```python
from build123d import *

# Parameters (mm, degrees)
F1_DEPTH       = 76.2
F1_DEPTH_BACK  = 76.2
F3_D           = 3.683
F3_CSINK_D     = 5.588
F3_CSINK_ANGLE = 100


with BuildPart() as f1:
    # F0 (on Front) → F1 (new body, two sides)
    with BuildSketch(Plane.XZ) as f1_sk:
        with BuildLine():
            Line((0, 1.0668), (0, 0))
            Line((0, 0), (127, 0))
            ThreePointArc((127, 0), (135.980256, -3.719744), (139.7, -12.7))
            Line((139.7, -12.7), (140.7668, -12.7))
            ThreePointArc((140.7668, -12.7), (136.734598, -2.965402), (127, 1.0668))
            Line((127, 1.0668), (0, 1.0668))
        make_face()
    extrude(amount=F1_DEPTH)
    extrude(f1_sk.sketch, amount=-F1_DEPTH_BACK)

    # F3 (through all)
    with Locations(Plane(origin=(0, 0, 0), x_dir=(1, 0, 0), z_dir=(0, 0, -1))):
        with Locations((63.5, 42.8625), (63.5, 0), (63.5, -42.8625)):
            CounterSinkHole(F3_D / 2, F3_CSINK_D / 2, counter_sink_angle=F3_CSINK_ANGLE)


solid = f1.part
```
Can you work these out from the model? Positions are in its coordinate system, mm. A direction names the side the tool comes from. Give positions to 0.01 mm unless a question says otherwise; leave off trailing zeros. Write each loop counter-clockwise with the first axis right and the second up, starting at its lowest first coordinate (ties: lowest second). Pieces come first, ordered by that corner, then holes. Notation, with made-up numbers: (-13, 79.5) -> (15, 79.5) arc R18 ccw to (15, 114.5) -> close; hole circle Ø8 at (-38, 81). An arc over 180 degrees is marked (long way). One line per item, written item: value.
Q1. Imagine slicing it at B-B on y = 0. Please give me the cut outline in (x, z), and give its area (3 significant figures).
Results found:
outline: (0, 0) -> (60.71, 0) -> (61.66, 0.8) -> (61.66, 1.07) -> (0, 1.07) -> close; (65.34, 0.8) -> (66.29, 0) -> (127, 0) arc R12.7 cw to (139.7, -12.7) -> (140.77, -12.7) arc R13.77 ccw to (127, 1.07) -> (65.34, 1.07) -> close
area: 153 mm^2
Q2. Imagine slicing it at A-A on x = 63.5. Please give me the cut outline in (y, z).
Results found:
outline: (-76.2, 0) -> (-45.66, 0) -> (-44.7, 0.8) -> (-44.7, 1.07) -> (-76.2, 1.07) -> close; (-41.02, 0.8) -> (-40.07, 0) -> (-2.79, 0) -> (-1.84, 0.8) -> (-1.84, 1.07) -> (-41.02, 1.07) -> close; (1.84, 0.8) -> (2.79, 0) -> (40.07, 0) -> (41.02, 0.8) -> (41.02, 1.07) -> (1.84, 1.07) -> close; (44.7, 0.8) -> (45.66, 0) -> (76.2, 0) -> (76.2, 1.07) -> (44.7, 1.07) -> close
Q3. Imagine slicing it at C-C on y = 58. Please give me the cut outline in (x, z), and give its area (3 significant figures).
Results found:
outline: (0, 0) -> (127, 0) arc R12.7 cw to (139.7, -12.7) -> (140.77, -12.7) arc R13.77 ccw to (127, 1.07) -> (0, 1.07) -> close
area: 158 mm^2
Q4. For P1, Ø5, axis at x = 94, y = -60, coming from the -Z side; P2, Ø2, axis at x = 63.5, y = 0, coming from the +Z side; P3, Ø1.5, axis at y = 41.5, z = -4.5, coming from the +X side; P4, Ø4, axis at x = 63.5, y = -42.86, coming from the -Z side, each with a flat end and sliding along its axis, tell me the tip position at first contact or that it passes through.
Results found:
P1: stops at z = 0
P2: passes through
P3: stops at x = 138.58
P4: stops at z = 0.66
Q5. Imagine slicing it at D-D on x = 80. Please give me the cut outline in (y, z), and give its area (3 significant figures).
Results found:
outline: (-76.2, 0) -> (76.2, 0) -> (76.2, 1.07) -> (-76.2, 1.07) -> close
area: 163 mm^2
Q6. Please list where these lines run through material, in increasing order: line 1 (Y direction, x = 63.5, z = 0.9); line 2 (Z direction, x = 51.5, y = 67.5); line 3 (X direction, y = 13.5, z = -11.75). Write a range as [from, to].
Results found:
line 1: y = [-76.2, -44.7], [-41.02, -1.84], [1.84, 41.02], [44.7, 76.2]
line 2: z = [0, 1.07]
line 3: x = [139.66, 140.73]
Q7. Which directions (+Z, -Z, +X, -X, +Y, -Y) give clear straight access to the entire face, cutting with the end or side of a thin tool? Please do faces 1 (the face through (48, -1, 0)), 2 (the face through (136.84, -1.07, -3.07)).
Results found:
face 1: -Z, -X, +Y, -Y
face 2: +Z, +X, +Y, -Y
